Geometry check sheet. Reference: drawing and pictorial views, mm from the part's lowest x, y, z. A direction names the side the tool comes from. Give positions to 0.01 mm unless a question says otherwise; leave off trailing zeros. Write each loop counter-clockwise with the first axis right and the second up, starting at its lowest first coordinate (ties: lowest second). Pieces come first, ordered by that corner, then holes. Notation, with made-up numbers: M 14,-34.75 L 45,-34.75 A21 cw 45,-4.75 Z; hole C 34.5,-4 d10. An arc over 180 degrees is marked long. One line per item, written item: value. Start each with the question number.
1. Cross-section at A-A on z = 22.5. Record the cut outline in (x, y), then the cut area to 3 significant figures.
2. Gauge pin test, flat ends, axial feed: pin 1 (2 mm diameter, centred on y = 2.5, z = 1, fed in from -X); pin 2 (2.5 mm diameter, centred on x = 5, y = 18, fed in from +Z); pin 3 (2 mm diameter, centred on y = 2.5, z = 78.5, fed in from +X). Record the tip position at first contact, or that the pin passes through.
3. Release check for a two-part mould opening along X. For the marked faces 3, 4 and 5 record: pulls with the +X half, pulls with the -X half, needs draft (parallel to the pull), parting line crosses it, or undercut.
4. Scan lines: line 1 (X direction, y = 1, z = 5); line 2 (Z direction, x = 30, y = 4); line 3 (Z direction, x = 135, y = 1.1). Record each from-to range of solid material in increasing order.
5. Tool access check on the marked faces 1 and 2. Record the directions out of +Z, -Z, +X, -X, +Y, -Y that give a thin tool (end or side, any length) a straight path to the whole face; none if there is none.
6. Cross-section at B-B on x = 98.5. Record the cut outline in (y, z), then the cut area to 3 significant figures.
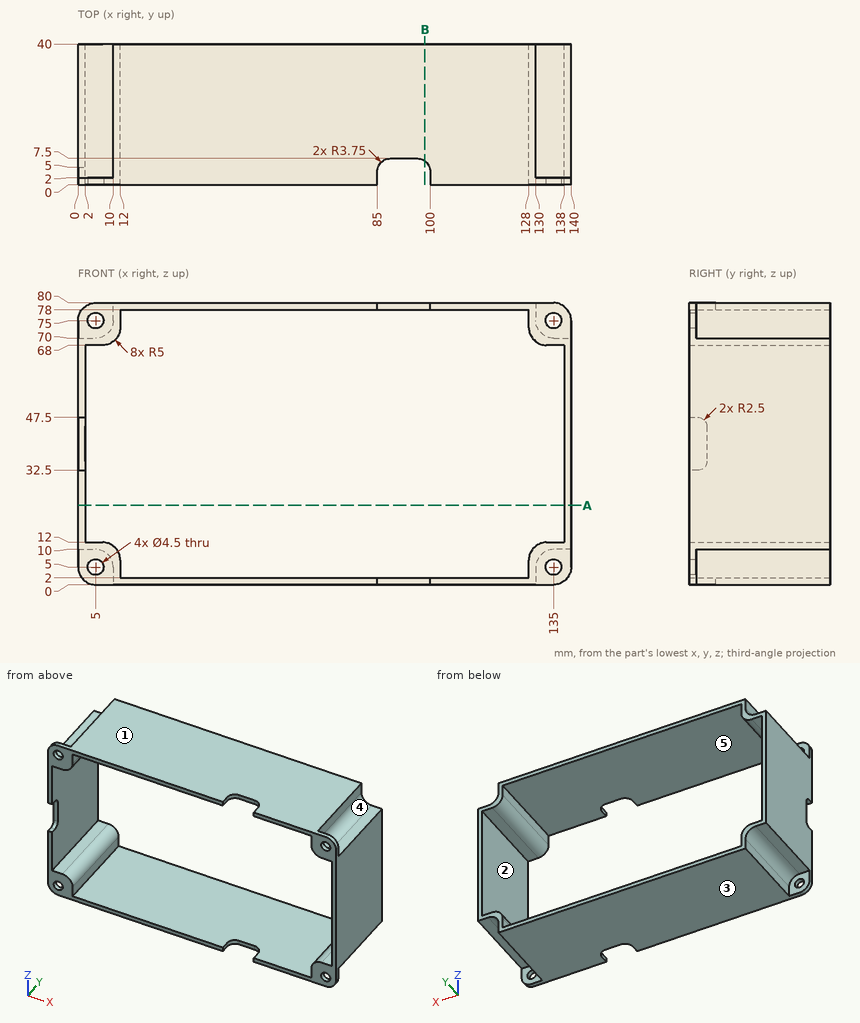
Report:
1. outline: M 0,0 L 2,0 L 2,40 L 0,40 Z; M 138,0 L 140,0 L 140,40 L 138,40 Z
1. area: 160 mm^2
2. pin 1: stops at x = 1.1
2. pin 2: stops at z = 70.16
2. pin 3: stops at x = 139.25
3. face 3: needs draft
3. face 4: pulls with the +X half
3. face 5: undercut
4. line 1: x = 0 to 2.75, 7.25 to 12, 128 to 132.75, 137.25 to 140
4. line 2: z = 0 to 2, 78 to 80
4. line 3: z = 0 to 2.75, 7.25 to 12, 68 to 72.75, 77.25 to 80
5. face 1: +Z, +X, -X, +Y, -Y
5. face 2: +Y, -Y
6. outline: M 6.75,0 L 40,0 L 40,2 L 6.75,2 Z; M 6.75,78 L 40,78 L 40,80 L 6.75,80 Z
6. area: 133 mm^2
